Design review of the part shown in the three views and the two pictorial views. Dimensions are in mm from the part's minimum x, y and z. A direction names the side the tool comes from. Coordinates: 2 decimals unless noted, no trailing zeros. Loops run counter-clockwise (first coordinate to the right, second up) from the corner with the lowest first, then second, coordinate; pieces in that order, holes last. Notation, with made-up numbers: (46, 82.5) -> (52, 82.5) arc R14 ccw to (52, 109.5) -> close; hole circle Ø11 at (36.25, -34.75). An arc over 180 degrees is marked (long way). Answer in a Markdown table with one row per item.
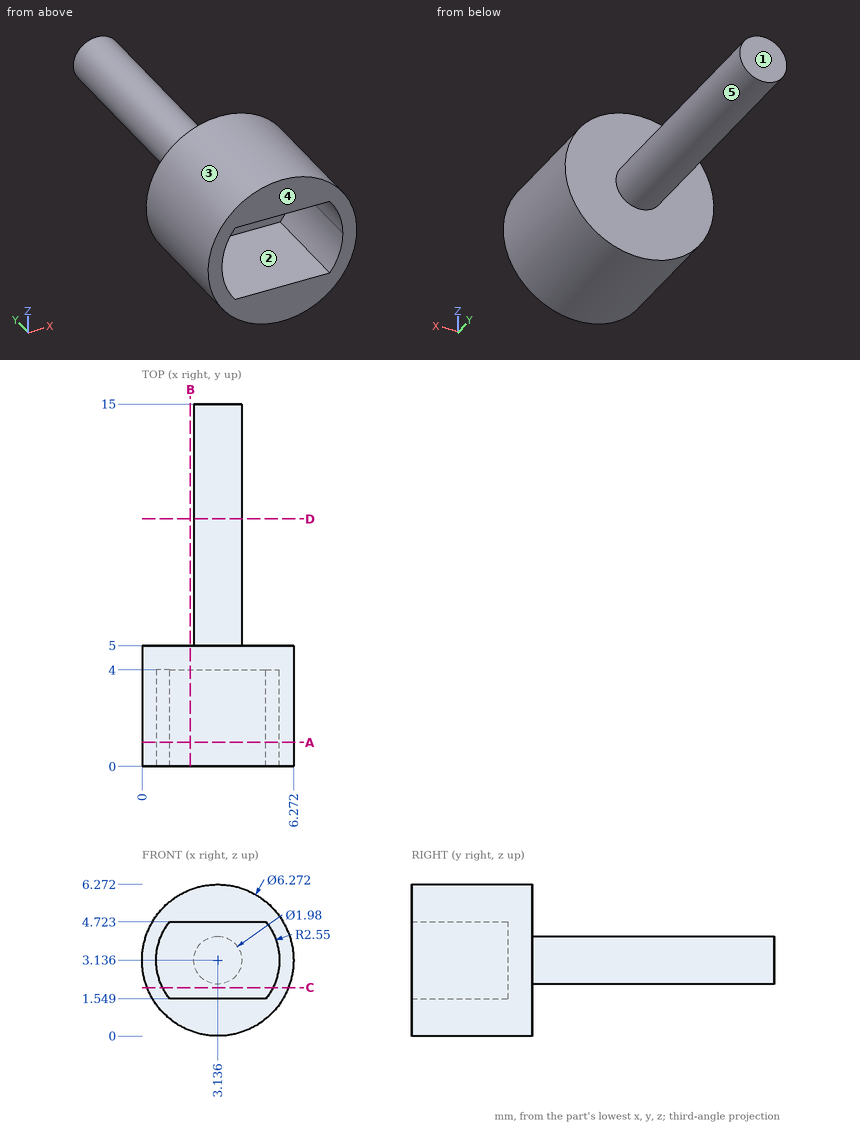
(1) Take a section at B-B on x = 2. Give the boundary of the cut face in (y, z).
Evaluation:
| item | result |
|---|---|
| outline | (0, 0.21) -> (5, 0.21) -> (5, 6.06) -> (0, 6.06) -> (0, 4.72) -> (4, 4.72) -> (4, 1.55) -> (0, 1.55) -> close |
(2) Take a section at D-D on y = 10.25. Give the boundary of the cut face in (x, z).
Evaluation:
| item | result |
|---|---|
| outline | circle Ø1.98 at (3.14, 3.14) |
(3) Take a section at C-C on z = 2. Give the boundary of the cut face in (x, y).
Evaluation:
| item | result |
|---|---|
| outline | (0.21, 0) -> (0.85, 0) -> (0.85, 4) -> (5.42, 4) -> (5.42, 0) -> (6.06, 0) -> (6.06, 5) -> (0.21, 5) -> close |
(4) Draft analysis for pull direction X (two halves, no side actions). For the marked faces 1, 2 and 3, state which applies: pulls with the +X half, pulls with the -X half, needs draft (parallel to the pull), parting line crosses it, or undercut.
Evaluation:
| item | result |
|---|---|
| face 1 | needs draft |
| face 2 | undercut |
| face 3 | parting line crosses it |
(5) To check wall thickness, follow probe 1 along Y at (x, z) = (2.75, 0.5); probe 2 along Y at (x, z) = (4, 2); probe 3 along Z at (x, y) = (2.5, 3) (1 decimal). State the ranges of each line that lie inside material, in increasing order.
Evaluation:
| item | result |
|---|---|
| probe 1 | y = 0 to 5 |
| probe 2 | y = 4 to 5 |
| probe 3 | z = 0.1 to 1.5, 4.7 to 6.2 |
(6) Tool access review of the marked faces 4 and 5: name each direction out of +Z, -Z, +X, -X, +Y, -Y from which nothing blocks a thin tool from reaching the whole face with its end or side.
Evaluation:
| item | result |
|---|---|
| face 4 | +Z, -Z, +X, -X, -Y |
| face 5 | +Y |
(7) For pin 1 (1 mm diameter, centred on x = 2, z = 3, fed in from +Y); pin 2 (2.5 mm diameter, centred on x = 3.5, z = 3, fed in from -Y), all flat-tipped, find the tip position at first contact; note any pin that passes through.
Evaluation:
| item | result |
|---|---|
| pin 1 | stops at y = 15 |
| pin 2 | stops at y = 4 |
(8) Take a section at A-A on y = 1. Give the boundary of the cut face in (x, z).
Evaluation:
| item | result |
|---|---|
| outline | circle Ø6.27 at (3.14, 3.14); hole (1.14, 1.55) -> (5.13, 1.55) arc R2.55 ccw to (5.13, 4.72) -> (1.14, 4.72) arc R2.55 ccw to start |
